```python
from build123d import *

# Parameters (mm, degrees)
F0_W     = 71
F0_H     = 100
F0_R     = 4.5
F1_DEPTH = 5
F2_W     = 5
F2_H     = 100
F3_DEPTH = 80
F4_R     = 6.25
F5_DEPTH = 71.001
F7_R     = 3
F8_DEPTH = 71.001


with BuildPart() as f1:
    # F0 (on Top) → F1 (new body)
    with BuildSketch(Plane.XY):
        with Locations((35.5, 0)):
            Rectangle(F0_W, F0_H)
        with Locations((52.5, 0)):
            Circle(F0_R, mode=Mode.SUBTRACT)
    extrude(amount=-F1_DEPTH)

    # F2 (on face) → F3 (join)
    with BuildSketch(Plane.XY):
        with Locations((29.5, 0)):
            Rectangle(F2_W, F2_H)
    extrude(amount=F3_DEPTH)

    # F4 (on Right) → F5 (cut, through all)
    with BuildSketch(Plane.YZ):
        with Locations((-27.5, 55)):
            Circle(F4_R)
        with Locations((27.5, 55)):
            Circle(F4_R)
    extrude(amount=F5_DEPTH, mode=Mode.SUBTRACT)

    # F6: F1 across face


with BuildPart() as f1_1:
    add(f1.part)
    add(f1.part.mirror(Plane(origin=(0, 0, -2.5), x_dir=(0, -1, 0), z_dir=(-1, 0, 0))))

    # F7 (on Right) → F8 (cut, through all)
    with BuildSketch(Plane.YZ):
        with Locations((-40, 70)):
            Circle(F7_R)
    extrude(amount=-F8_DEPTH, mode=Mode.SUBTRACT)


solid = f1_1.part
```
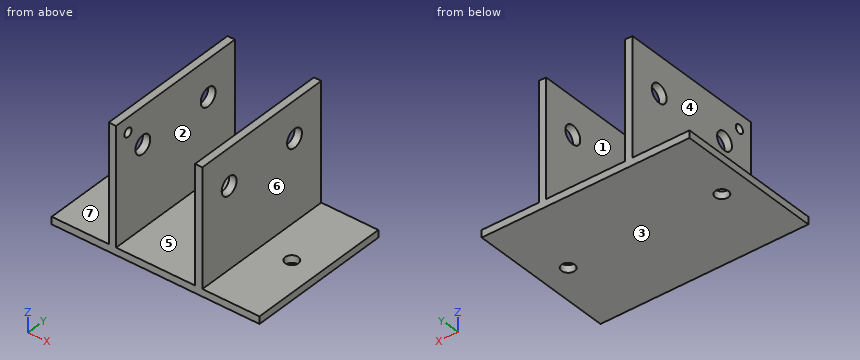
Geometry check sheet. Reference: the model listing, model coordinates, mm. Face numbers are marked on the shaded views. A direction names the side the tool comes from. Coordinates: 2 decimals unless noted, no trailing zeros. Write each loop counter-clockwise with the first axis right and the second up, starting at its lowest first coordinate (ties: lowest second). Pieces come first, ordered by that corner, then holes. Notation, with made-up numbers: M -12,12 L 38,12 A16 cw 38,41 Z; hole C 63.25,28 d2. An arc over 180 degrees is marked long. One line per item, written item: value. Start each with the question number.
(1) Release check for a two-part mould opening along X. For the marked faces 1, 2, 3 and 4 record: released by +X, released by -X, zero draft, split by the parting line, or undercut.
(2) Depth check by flat-ended pin: pin 1 (5 mm diameter, centred on y = -9.5, z = 29.5, fed in from -X); pin 2 (24 mm diameter, centred on y = -14.5, z = 24.5, fed in from +X). Enter the tip coordinate at first touch or a pass-through.
(3) Tool access check on the marked faces 5, 6 and 7. Record the directions out of +Z, -Z, +X, -X, +Y, -Y that give a thin tool (end or side, any length) a straight path to the whole face; none if there is none.
(4) Scan lines: line 1 along Y through (x, z) = (-30.7, 55); line 2 along X through (y, z) = (-22.5, 37); line 3 along Y through (x, z) = (-52.5, -2.3). Record each from-to range of solid material in increasing order. Write a range as [from, to].
(5) Sectioned sample at B-B, the plane y = -40. Enter the section's corners in (x, z).
(6) Sectioned sample at C-C, the plane x = -52.5. Enter the section's corners in (y, z).
(7) Sectioned sample at A-A, the plane z = 26. Enter the section's corners in (x, y).
(8) Sectioned sample at D-D, the plane y = 27.5. Enter the section's corners in (x, z), and give its area (4 significant figures).
Filled sheet:
1. face 1: undercut
1. face 2: undercut
1. face 3: zero draft
1. face 4: released by -X
2. pin 1: x = -32
2. pin 2: x = 32
3. face 5: +Z, +Y, -Y
3. face 6: +Z, +X, +Y, -Y
3. face 7: +Z, -X, +Y, -Y
4. line 1: [-50, -33.75], [-21.25, 21.25], [33.75, 50]
4. line 2: [-32, -27], [27, 32]
4. line 3: [-50, -4.5], [4.5, 50]
5. outline: M -71,-5 L 71,-5 L 71,0 L 32,0 L 32,80 L 27,80 L 27,0 L -27,0 L -27,67 L -32,67 L -32,0 L -71,0 Z; M -32,73 L -27,73 L -27,80 L -32,80 Z
6. outline: M -50,-5 L -4.5,-5 L -4.5,0 L -50,0 Z; M 4.5,-5 L 50,-5 L 50,0 L 4.5,0 Z
7. outline: M -32,-50 L -27,-50 L -27,50 L -32,50 Z; M 27,-50 L 32,-50 L 32,50 L 27,50 Z
8. outline: M -71,-5 L 71,-5 L 71,0 L 32,0 L 32,48.75 L 27,48.75 L 27,0 L -27,0 L -27,48.75 L -32,48.75 L -32,0 L -71,0 Z; M -32,61.25 L -27,61.25 L -27,80 L -32,80 Z; M 27,61.25 L 32,61.25 L 32,80 L 27,80 Z
8. area: 1,385 mm²
